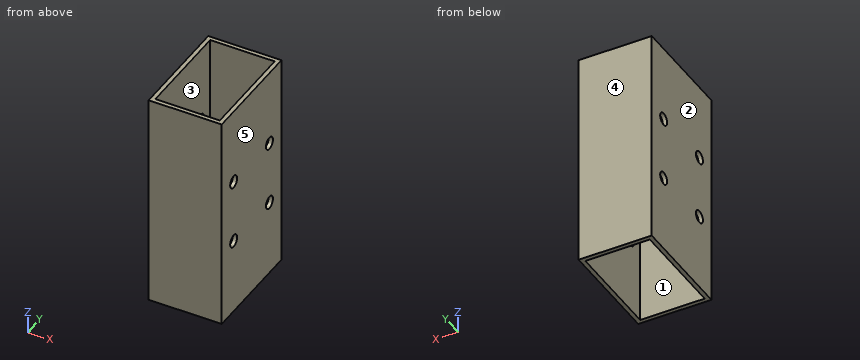
```python
from build123d import *

# Parameters (mm, degrees)
F0_W     = 17
F0_H     = 50.6
F1_DEPTH = 25
F2_T     = -1
F3_R     = 1.45
F4_DEPTH = 25


with BuildPart() as f1:
    # F0 (on Front) → F1 (new body)
    with BuildSketch(Plane.XZ):
        Rectangle(F0_W, F0_H)
    extrude(amount=F1_DEPTH)

    # F2
    f2_openings = [f1.faces().sort_by_distance(p)[0] for p in [
        (0, -12.5, 25.3),
        (0, -12.5, -25.3),
    ]]
    offset(amount=F2_T, openings=f2_openings)

    # F3 (on face) → F4 (cut)
    with BuildSketch(Plane.YZ.offset(8.5)):
        with Locations((-5, 7.5)):
            Circle(F3_R)
        with Locations((-20, 7.5)):
            Circle(F3_R)
        with Locations((-20, -7.5)):
            Circle(F3_R)
        with Locations((-5, -7.5)):
            Circle(F3_R)
    extrude(amount=-F4_DEPTH, mode=Mode.SUBTRACT)


solid = f1.part
```
CAD build for the part. Positions are in the model's coordinates, mm. Face numbers are marked on the shaded views. A direction names the side the tool comes from. Coordinates: 2 decimals unless noted, no trailing zeros. Order: outer loops, then holes, each group sorted by start corner. A loop starts at its lowest first (then second) coordinate and runs counter-clockwise, first axis right, second up. Notation, with made-up numbers: (46.25, -14.75) - (54.25, -14.75) arc R19 cw to (54.25, -6.75) - close; hole circle Ø7 at (-16, 84). An arc over 180 degrees is marked (long way). Use a Markdown table: item, result. Add a question column.
(1) Drill centre lines: line 1 along Z through (x, y) = (7.95, -20); line 2 along X through (y, z) = (-6.5, 9.5); line 3 along Y through (x, z) = (-3, -21). Where is each one in solid material? Low to high. Write a range as [from, to].
(2) Saw through at D-D (z = -14). Give the cut face in (x, y), then the cut area to 3 significant figures.
(3) Saw through at A-A (z = -7.5). Give the cut face in (x, y).
(4) Saw through at C-C (x = 7). Give the cut face in (y, z).
(5) Saw through at B-B (y = -5). Give the cut face in (x, z), then the cut area to 3 significant figures.
(6) Pull direction X, two halves, no side cores. Call the marked faces 3, 4 and 5: +X half, -X half, draft (parallel to the pull), parting line (faces both ways), or undercut.
(7) Which spindle directions (+Z, -Z, +X, -X, +Y, -Y) get a long thin tool onto all of the face, cutting with end or side? Do the marked faces 1 and 2. Say none if no direction does.
(8) Flat gauge pin, fed straight in: pin 1 (3.5 mm diameter, centred on y = -5, z = 7.5, fed in from +X). Where does the tip first touch, or does it go through?
Solved:
| question | item | result |
|---|---|---|
| 1 | line 1 | z = [-25.3, -8.95], [-6.05, 6.05], [8.95, 25.3] |
| 1 | line 2 | x = [-8.5, -7.5], [7.5, 8.5] |
| 1 | line 3 | y = [-25, -24], [-1, 0] |
| 2 | outline | (-8.5, -25) - (8.5, -25) - (8.5, 0) - (-8.5, 0) - close; hole (-7.5, -24) - (7.5, -24) - (7.5, -1) - (-7.5, -1) - close |
| 2 | area | 80.0 mm² |
| 3 | outline | (-8.5, -25) - (8.5, -25) - (8.5, -21.45) - (7.5, -21.45) - (7.5, -24) - (-7.5, -24) - (-7.5, -21.45) - (-8.5, -21.45) - close; (-8.5, -18.55) - (-7.5, -18.55) - (-7.5, -6.45) - (-8.5, -6.45) - close; (-8.5, -3.55) - (-7.5, -3.55) - (-7.5, -1) - (7.5, -1) - (7.5, -3.55) - (8.5, -3.55) - (8.5, 0) - (-8.5, 0) - close; (7.5, -18.55) - (8.5, -18.55) - (8.5, -6.45) - (7.5, -6.45) - close |
| 4 | outline | (-25, -25.3) - (-24, -25.3) - (-24, 25.3) - (-25, 25.3) - close; (-1, -25.3) - (0, -25.3) - (0, 25.3) - (-1, 25.3) - close |
| 5 | outline | (-8.5, -25.3) - (-7.5, -25.3) - (-7.5, -8.95) - (-8.5, -8.95) - close; (-8.5, -6.05) - (-7.5, -6.05) - (-7.5, 6.05) - (-8.5, 6.05) - close; (-8.5, 8.95) - (-7.5, 8.95) - (-7.5, 25.3) - (-8.5, 25.3) - close; (7.5, -25.3) - (8.5, -25.3) - (8.5, -8.95) - (7.5, -8.95) - close; (7.5, -6.05) - (8.5, -6.05) - (8.5, 6.05) - (7.5, 6.05) - close; (7.5, 8.95) - (8.5, 8.95) - (8.5, 25.3) - (7.5, 25.3) - close |
| 5 | area | 89.6 mm² |
| 6 | face 3 | undercut |
| 6 | face 4 | draft |
| 6 | face 5 | +X half |
| 7 | face 1 | +Z, -Z |
| 7 | face 2 | +Z, -Z, -X, +Y, -Y |
| 8 | pin 1 | stops at x = 8.5 |
